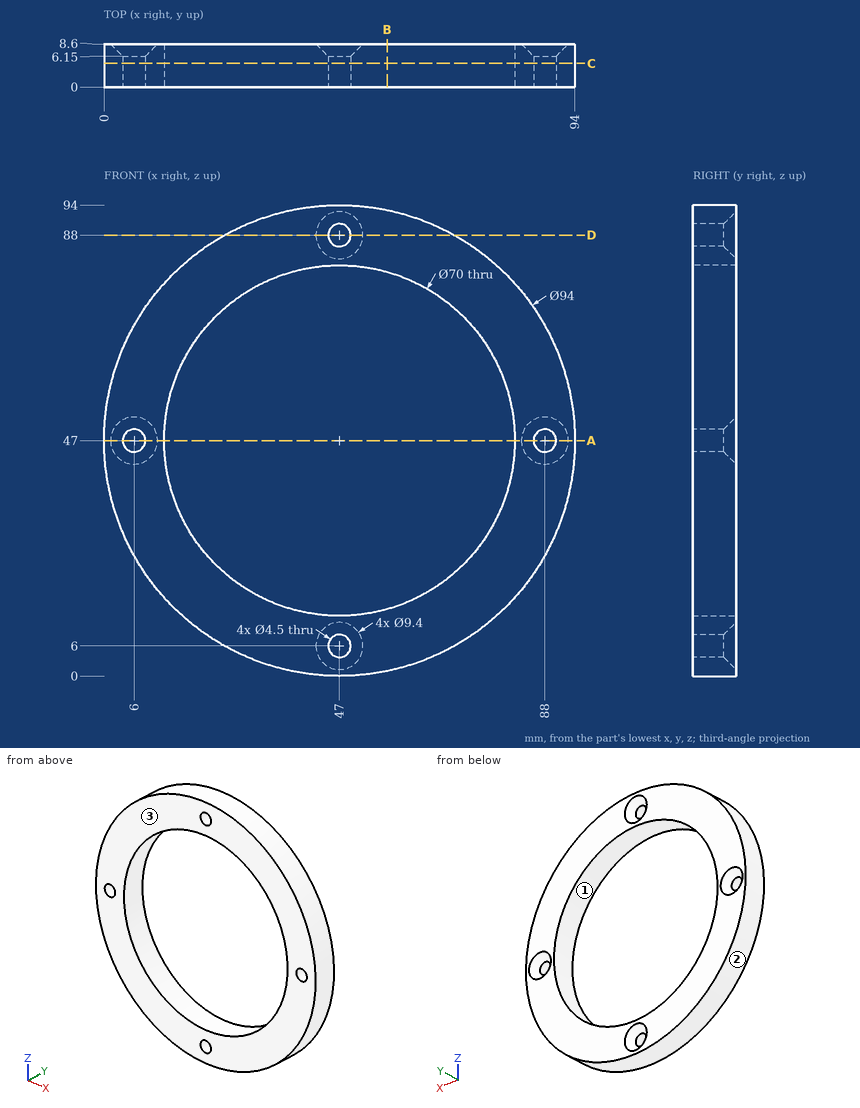
Could you check a few things on this drawing? It's one solid part, dimensions in mm from its lowest x, y, z. Coordinates: 2 decimals unless noted, no trailing zeros. Loops run counter-clockwise (first coordinate to the right, second up) from the corner with the lowest first, then second, coordinate; pieces in that order, holes last. Notation, with made-up numbers: (14.25, 59.25) - (26.25, 59.25) arc R33 cw to (26.25, 92.25) - close; hole circle Ø1 at (43.5, 13.25). An arc over 180 degrees is marked (long way). Return JSON: item names as keys, results as strings. Group by question number.
Item 1: I need wall thicknesses on line 1 (X direction, y = 1.5, z = 47); line 2 (X direction, y = 6.25, z = 49); line 3 (Z direction, x = 86, y = 3). Which ranges of each line are inside material? Lowest first, please. Write a range as from..to.
Item 2: If we section it at B-B on x = 56.5: Write out the boundary of the cut face in (y, z), and give its area (3 significant figures).
Item 3: We'd pull the mould along Z, two halves only. Please class the marked faces 1, 2 and 3: +Z half, -Z half, draft (parallel to the pull), parting line (faces both ways), or undercut.
Item 4: If we section it at C-C on y = 4.75: Write out the boundary of the cut face in (x, z).
Item 5: If we section it at D-D on z = 88: Write out the boundary of the cut face in (x, y).
Item 6: If we section it at A-A on z = 47: Write out the boundary of the cut face in (x, y).
Item 7: Will these pins go through, and if not, where does the flat tip stop? P1, Ø3, axis at y = 2.5, z = 41.5, coming from the -X side; P2, Ø6, axis at x = 47, z = 6, coming from the +Y side; P3, Ø5, axis at y = 4, z = 36, coming from the +X side (3 decimals).
Calculated:
{
 "1": {"line 1": "x = 0..3.75, 8.25..12, 82..85.75, 90.25..94", "line 2": "x = 0.04..4.77, 7.23..12.06, 81.94..86.77, 89.23..93.96", "line 3": "z = 20.77..45.97, 48.03..73.23"},
 "2": {"outline": "(0, 0.97) - (8.6, 0.97) - (8.6, 13.31) - (0, 13.31) - close; (0, 80.69) - (8.6, 80.69) - (8.6, 93.03) - (0, 93.03) - close", "area": "212 mm^2"},
 "3": {"face 1": "undercut", "face 2": "parting line", "face 3": "draft"},
 "4": {"outline": "circle Ø94 at (47, 47); hole circle Ø4.5 at (6, 47); hole circle Ø70 at (47, 47); hole circle Ø4.5 at (47, 6); hole circle Ø4.5 at (47, 88); hole circle Ø4.5 at (88, 47)"},
 "5": {"outline": "(24.02, 0) - (44.75, 0) - (44.75, 6.15) - (42.3, 8.6) - (24.02, 8.6) - close; (49.25, 0) - (69.98, 0) - (69.98, 8.6) - (51.7, 8.6) - (49.25, 6.15) - close"},
 "6": {"outline": "(0, 0) - (3.75, 0) - (3.75, 6.15) - (1.3, 8.6) - (0, 8.6) - close; (8.25, 0) - (12, 0) - (12, 8.6) - (10.7, 8.6) - (8.25, 6.15) - close; (82, 0) - (85.75, 0) - (85.75, 6.15) - (83.3, 8.6) - (82, 8.6) - close; (90.25, 0) - (94, 0) - (94, 8.6) - (92.7, 8.6) - (90.25, 6.15) - close"},
 "7": {"P1": "stops at x = 0.17", "P2": "stops at y = 6.9", "P3": "stops at x = 93.225"}
}
